```python
from build123d import *

# Parameters (mm, degrees)
F1_DEPTH = 101.6
F0_W     = 203.2
F0_H     = 88.9
F2_DEPTH = 25.4


with BuildPart() as f1:
    # F0 (on Front) → F1 (new body, symmetric)
    with BuildSketch(Plane.XZ):
        Polygon((101.6, -1003.3), (101.6, 901.7), (-101.6, 827.9892), (-101.6, -1003.3), align=None)
    extrude(amount=F1_DEPTH, both=True)

    # F0 (on Front) → F2 (join, symmetric)
    with BuildSketch(Plane.XZ):
        Polygon((71.284475, 985.2714), (-101.6, 922.557557), (-101.6, 827.9892), (101.6, 901.7), align=None)
        with Locations((0, -1047.75)):
            Rectangle(F0_W, F0_H)
    extrude(amount=F2_DEPTH, both=True)


solid = f1.part
```
For this review, take the finished solid that the model builds, in its own axes (mm). A direction names the side the tool comes from. Coordinates: 2 decimals unless noted, no trailing zeros. Write each loop counter-clockwise with the first axis right and the second up, starting at its lowest first coordinate (ties: lowest second). Pieces come first, ordered by that corner, then holes. Notation, with made-up numbers: (21, -8) -> (52, -8) arc R16 ccw to (52, 6) -> close; hole circle Ø2 at (-29.75, 76.5). An arc over 180 degrees is marked (long way). Put each result on its own line as item: value.
Q1. Tool access review of faces 1 (the flat face through (-1, 25.4, 908)), 2 (the flat face through (1.42, -64.03, 865.36)), 3 (the flat face through (-1, 25.4, -1047)), 4 (the flat face through (-13.948, 0.356, 954.353)), 5 (the flat face through (-1, -64, -1003.3)): name each direction out of +Z, -Z, +X, -X, +Y, -Y from which nothing blocks a thin tool from reaching the whole face with its end or side.
From the geometry:
face 1: +Z, -X, +Y
face 2: +Z, -X, -Y
face 3: -Z, +X, -X, +Y
face 4: +Z, -X, +Y, -Y
face 5: -Z, +X, -X, -Y
Q2. Take a section at B-B, the plane x = 21.5. State the section outline as (y, z) points.
From the geometry:
outline: (-101.6, -1003.3) -> (-25.4, -1003.3) -> (-25.4, -1092.2) -> (25.4, -1092.2) -> (25.4, -1003.3) -> (101.6, -1003.3) -> (101.6, 872.64) -> (25.4, 872.64) -> (25.4, 967.21) -> (-25.4, 967.21) -> (-25.4, 872.64) -> (-101.6, 872.64) -> close
Q3. Take a section at A-A, the plane y = 6. State the section outline as (x, z) points, then the cut area to 3 significant figures.
From the geometry:
outline: (-101.6, -1092.2) -> (101.6, -1092.2) -> (101.6, 901.7) -> (71.28, 985.27) -> (-101.6, 922.56) -> close
area: 415,000 mm2
Q4. Wall thickness on L1, parallel to Z at x = -6, y = 74.5; L2, parallel to Z at x = 49, y = -81: over which ranges is each line inside the solid? List them lowest first.
From the geometry:
L1: z = -1003.3 to 862.67
L2: z = -1003.3 to 882.62
Q5. Clearance check with flat-ended pins moving along their axes: pin 1 Ø1 at (x, y) = (-53.5, 63) entering from -Z; pin 2 Ø12 at (x, y) = (13, 52.5) entering from +Z; pin 3 Ø5 at (x, y) = (-13, -47.5) entering from +Z. State where each tip first meets the part, or that it passes through.
From the geometry:
pin 1: stops at z = -1003.3
pin 2: stops at z = 871.74
pin 3: stops at z = 861.04
Q6. Take a section at C-C, the plane y = 82.5. State the section outline as (x, z) points, then the cut area to 3 significant figures.
From the geometry:
outline: (-101.6, -1003.3) -> (101.6, -1003.3) -> (101.6, 901.7) -> (-101.6, 827.99) -> close
area: 380,000 mm2
